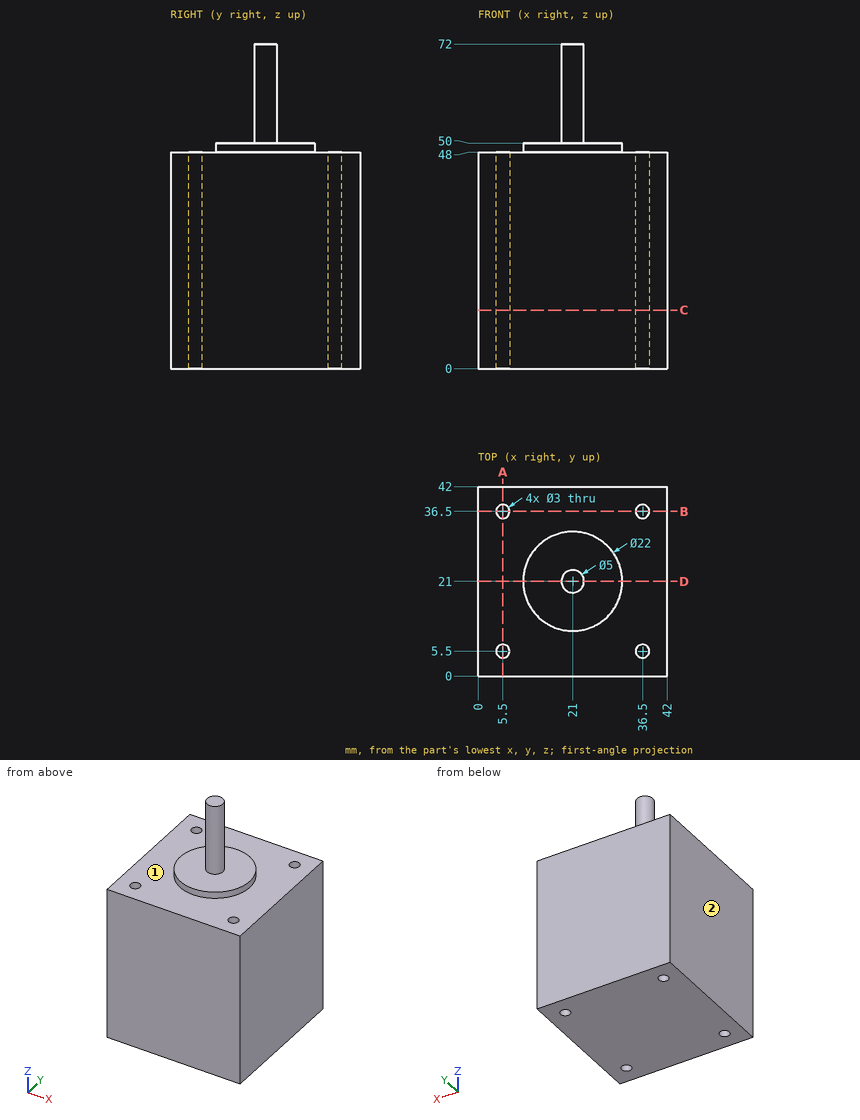
Design review of the part shown in the three views and the two pictorial views. Dimensions are in mm from the part's minimum x, y and z. A direction names the side the tool comes from. Round coordinates to 2 decimals unless told otherwise and drop trailing zeros. Order: outer loops, then holes, each group sorted by start corner. A loop starts at its lowest first (then second) coordinate and runs counter-clockwise, first axis right, second up.
Item 1: For pin 1 (12 mm diameter, centred on x = 9.5, z = 63.5, fed in from -Y); pin 2 (5 mm diameter, centred on x = 5.5, y = 36.5, fed in from +Z), all flat-tipped, find the tip position at first contact; note any pin that passes through.
Working result:
pin 1: passes through
pin 2: stops at z = 48
Item 2: Add section C-C, the plane z = 13. State the section outline as (x, y) points, and give its area (3 significant figures).
Working result:
outline: (0, 0) - (42, 0) - (42, 42) - (0, 42) - close; hole circle Ø3 at (5.5, 5.5); hole circle Ø3 at (5.5, 36.5); hole circle Ø3 at (36.5, 5.5); hole circle Ø3 at (36.5, 36.5)
area: 1,740 mm2
Item 3: Add section D-D, the plane y = 21. State the section outline as (x, z) points.
Working result:
outline: (0, 0) - (42, 0) - (42, 48) - (32, 48) - (32, 50) - (23.5, 50) - (23.5, 72) - (18.5, 72) - (18.5, 50) - (10, 50) - (10, 48) - (0, 48) - close
Item 4: Machinability: for the marked faces 1 and 2, which of the approach directions +Z, -Z, +X, -X, +Y, -Y give a long, thin tool a straight path to every point of the face, cutting with its end or side? Answer none if there is none.
Working result:
face 1: +Z
face 2: +Z, -Z, -X, +Y, -Y
Item 5: To check wall thickness, follow probe 1 along Y at (x, z) = (5.5, 25.5); probe 2 along X at (y, z) = (5, 19). State the ranges of each line that lie inside material, in increasing order.
Working result:
probe 1: y = 0 to 4, 7 to 35, 38 to 42
probe 2: x = 0 to 4.09, 6.91 to 35.09, 37.91 to 42
Item 6: Add section A-A, the plane x = 5.5. State the section outline as (y, z) points, and give its area (3 significant figures).
Working result:
outline: (0, 0) - (4, 0) - (4, 48) - (0, 48) - close; (7, 0) - (35, 0) - (35, 48) - (7, 48) - close; (38, 0) - (42, 0) - (42, 48) - (38, 48) - close
area: 1,730 mm2
